from build123d import *

# Parameters (mm, degrees)
SKETCH1_R           = 3
BOSS_EXTRUDE1_DEPTH = 22.5
SKETCH3_W           = 60
SKETCH3_H           = 30
CUT_EXTRUDE1_DEPTH  = 121.959704034
FILLET1_R           = 10
CUT_EXTRUDE2_DEPTH  = 30
CUT_EXTRUDE4_DEPTH  = 30
FILLET2_R           = 10
SKETCH6_R           = 6.1
CUT_EXTRUDE5_DEPTH  = 3.2
CUT_EXTRUDE6_START  = -3.2
SKETCH7_R           = 6.1
CUT_EXTRUDE6_DEPTH  = 3.2


with BuildPart() as part:
    # Sketch1 → Boss-Extrude1 (new, symmetric)
    with BuildSketch(Plane.XY):
        with BuildLine():
            Line((-100, -15), (100, -15))
            ThreePointArc((100, -15), (115, 0), (100, 15))
            Line((100, 15), (-100, 15))
            Line((-100, 15), (-100, -15))
        make_face()
        with Locations(Location((-80, 0, 0), (0, 0, 180))):
            Circle(SKETCH1_R, mode=Mode.SUBTRACT)
    extrude(amount=BOSS_EXTRUDE1_DEPTH, both=True)

    # Sketch3 → Cut-Extrude1 (cut, through all)
    with BuildSketch(Plane(origin=(0, 15, 0), x_dir=(1, 0, 0), z_dir=(0, 1, 0))):
        with Locations((-70, 0)):
            Rectangle(SKETCH3_W, SKETCH3_H)
    extrude(amount=-CUT_EXTRUDE1_DEPTH, mode=Mode.SUBTRACT)

    # Fillet1
    fillet1_edges = [part.edges().sort_by_distance(p)[0] for p in [
        (-100, -15, -18.75),
        (-100, 15, -18.75),
        (-100, -15, 18.75),
        (-100, 15, 18.75),
    ]]
    fillet(fillet1_edges, radius=FILLET1_R)

    # Sketch4 → Cut-Extrude2 (cut)
    with BuildSketch(Plane(origin=(0, 0, -15), x_dir=(-1, 0, 0), z_dir=(0, 0, -1))):
        Polygon((40, 15), (40, 0), (10, 15), align=None)
    extrude(amount=-CUT_EXTRUDE2_DEPTH, mode=Mode.SUBTRACT)

    # Sketch5 → Cut-Extrude4 (cut)
    with BuildSketch(Plane(origin=(0, 0, -15), x_dir=(-1, 0, 0), z_dir=(0, 0, -1))):
        Polygon((40, 0), (40, -15), (10, -15), align=None)
    extrude(amount=-CUT_EXTRUDE4_DEPTH, mode=Mode.SUBTRACT)

    # Fillet2
    fillet2_edges = [part.edges().sort_by_distance(p)[0] for p in [
        (-40, 0, 0),
    ]]
    fillet(fillet2_edges, radius=FILLET2_R)

    # Sketch6 → Cut-Extrude5 (cut)
    with BuildSketch(Plane.XY.offset(22.5)):
        with Locations((-80, 0)):
            Circle(SKETCH6_R)
    extrude(amount=-CUT_EXTRUDE5_DEPTH, mode=Mode.SUBTRACT)

    # Sketch7 → Cut-Extrude6 (cut)
    with BuildSketch(Plane(origin=(0, 0, -22.5), x_dir=(-1, 0, 0), z_dir=(0, 0, -1)).offset(CUT_EXTRUDE6_START)):
        with Locations(Location((80, 0, 0), (0, 0, 180))):
            Circle(SKETCH7_R)
    extrude(amount=CUT_EXTRUDE6_DEPTH, mode=Mode.SUBTRACT)


solid = part.part
Part model, mm, in its own coordinate system. A direction names the side the tool comes from. Give positions to 0.01 mm unless a question says otherwise; leave off trailing zeros. Order: outer loops, then holes, each group sorted by start corner. A loop starts at its lowest first (then second) coordinate and runs counter-clockwise, first axis right, second up. Notation, with made-up numbers: (-20, 41) - (-14, 41) arc R29 ccw to (-14, 72) - close; hole circle Ø9 at (71.5, -31). An arc over 180 degrees is marked (long way). One line per question, with ' | ' between items.
1. Band-saw the part on B-B on z = 17. List the corners of the cut face in (x, y).
Filled in:
outline: (-100, -5) arc R10 ccw to (-90, -15) - (100, -15) arc R15 ccw to (100, 15) - (-90, 15) arc R10 ccw to (-100, 5) - close; hole circle Ø6 at (-80, 0)
2. Band-saw the part on D-D on z = 6.5. List the corners of the cut face in (x, y), then the cut area to 3 significant figures.
Filled in:
outline: (-22.11, -8.94) - (-10, -15) - (100, -15) arc R15 ccw to (100, 15) - (-10, 15) - (-22.11, 8.94) arc R10 ccw to start | area: 4,010 mm²
3. Drop flat-ended pins along their axis: P1, Ø6, axis at x = -79.5, y = 1.5, coming from the -Z side; P2, Ø3.5, axis at x = -78, y = 1.5, coming from the +Z side; P3, Ø1, axis at y = -1.5, z = 10.5, coming from the -X side. Give the stop position or say it passes through.
Filled in:
P1: z = -19.3 | P2: z = 19.3 | P3: x = -27.59
4. Which spindle directions (+Z, -Z, +X, -X, +Y, -Y) get a long thin tool onto all of the face, cutting with end or side? Do faces 5 (the face through (-74.365, 2.336, -20.878)), 6 (the face through (-97.15, 11.99, 18.7)), 7 (the face through (-27.64, -0.15, 0.21)), 8 (the face through (-83, -1, 19.3)). Say none if no direction does.
Filled in:
face 5: -Z | face 6: +Z, -Z, -X, +Y | face 7: -X | face 8: +Z
5. Band-saw the part on A-A on x = -56. List the corners of the cut face in (y, z), then the cut area to 3 significant figures.
Filled in:
outline: (-15, -22.5) - (15, -22.5) - (15, -15) - (-15, -15) - close; (-15, 15) - (15, 15) - (15, 22.5) - (-15, 22.5) - close | area: 450 mm²
6. Drill centre lines: probe 1 along Y at (x, z) = (-80, 20.3); probe 2 along Y at (x, z) = (-80, -18.4); probe 3 along Z at (x, y) = (-81.5, 12). Where is each one in solid material? Low to high.
Filled in:
probe 1: -15 to -6.1, 6.1 to 15 | probe 2: -15 to -3, 3 to 15 | probe 3: -22.5 to -15, 15 to 22.5
7. Pull direction Z, two halves, no side cores. Call faces 1 (the face through (6, 0, 22.5)), 2 (the face through (-83, 1, -19.3)), 3 (the face through (-77, 0, 17)), 4 (the face through (-16, -12, 0)): +Z half, -Z half, draft (parallel to the pull), parting line (faces both ways), or undercut.
Filled in:
face 1: +Z half | face 2: -Z half | face 3: draft | face 4: undercut
8. Band-saw the part on C-C on x = -80. List the corners of the cut face in (y, z), then the cut area to 3 significant figures.
Filled in:
outline: (-15, -22.5) - (-6.1, -22.5) - (-6.1, -19.3) - (-3, -19.3) - (-3, -15) - (-15, -15) - close; (-15, 15) - (-3, 15) - (-3, 19.3) - (-6.1, 19.3) - (-6.1, 22.5) - (-15, 22.5) - close; (3, -19.3) - (6.1, -19.3) - (6.1, -22.5) - (15, -22.5) - (15, -15) - (3, -15) - close; (3, 15) - (15, 15) - (15, 22.5) - (6.1, 22.5) - (6.1, 19.3) - (3, 19.3) - close | area: 320 mm²
